Work out the finished part from the listing and answer in its coordinate system (mm). Face numbers are marked on the shaded views. Round coordinates to 2 decimals unless told otherwise and drop trailing zeros. Loops run counter-clockwise (first coordinate to the right, second up) from the corner with the lowest first, then second, coordinate; pieces in that order, holes last. Notation, with made-up numbers: M 40,86.25 L 80,86.25 A9 cw 80,93.25 Z; hole C 68,-37.75 d4. An arc over 180 degrees is marked long. One line per item, written item: value.
```python
from build123d import *

# Parameters (mm, degrees)
SKETCH024_R     = 47.5
PAD007_DEPTH    = 5
SKETCH025_W     = 13.5
SKETCH025_H     = 46
POCKET014_DEPTH = 2.5
SKETCH026_R     = 1.75
POCKET015_DEPTH = 5
SKETCH023_W     = 13.2
SKETCH023_H     = 2.5
PAD008_DEPTH    = 1


with BuildPart() as part:
    # Sketch024 → Pad007 (new body)
    with BuildSketch(Plane.XY):
        Circle(SKETCH024_R)
    extrude(amount=PAD007_DEPTH)

    # Sketch025 (on Face3 of Pad007) → Pocket014 (cut)
    with BuildSketch(Plane.XY.offset(5)):
        Rectangle(SKETCH025_W, SKETCH025_H)
    extrude(amount=-POCKET014_DEPTH, mode=Mode.SUBTRACT)

    # Sketch026 (on Face3 of Pocket014) → Pocket015 (cut)
    with BuildSketch(Plane.XY.offset(5)):
        with Locations((-40, 0)):
            Circle(SKETCH026_R)
        with Locations((-12.363995, 38.041183)):
            Circle(SKETCH026_R)
        with Locations((32.356581, 23.51705)):
            Circle(SKETCH026_R)
        with Locations((32.366826, -23.502949)):
            Circle(SKETCH026_R)
        with Locations((-12.347418, -38.046567)):
            Circle(SKETCH026_R)
    extrude(amount=-POCKET015_DEPTH, mode=Mode.SUBTRACT)

    # Sketch023 (on Face3 of Pocket015) → Pad008 (join)
    with BuildSketch(Plane.XY.offset(5)):
        with Locations((0, 34.25)):
            Rectangle(SKETCH023_W, SKETCH023_H)
    extrude(amount=PAD008_DEPTH)


solid = part.part
```
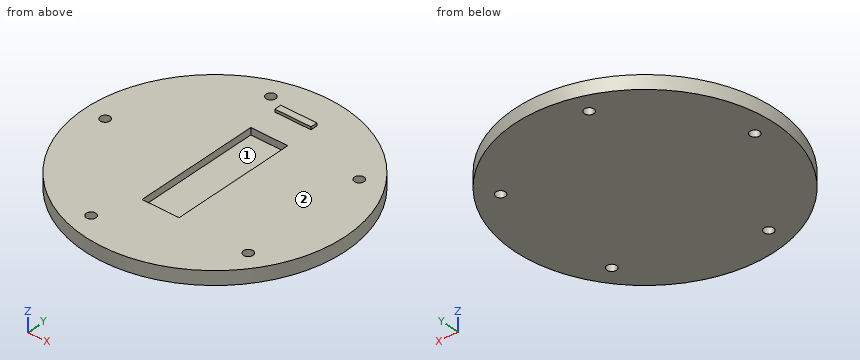
1) Each of these flat-tipped pins is pushed along its axis until it touches: pin 1 (0.8 mm diameter, centred on x = -3, z = 4.5, fed in from +Y); pin 2 (1.2 mm diameter, centred on y = 10.5, z = 3.5, fed in from -X); pin 3 (3 mm diameter, centred on x = 32.37, y = -23.5, fed in from +Z); pin 4 (7 mm diameter, centred on x = 1, y = -1.5, fed in from +Z). Where does it stop, or does it pass through?
Check values:
pin 1: y = 47.43
pin 2: x = -46.46
pin 3: through
pin 4: z = 2.5
2) Find section B-B (x = -40). Give the vertices of the cut face in (y, z), then the cut area to 3 significant figures.
Check values:
outline: M -25.62,0 L -1.75,0 L -1.75,5 L -25.62,5 Z; M 1.75,0 L 25.62,0 L 25.62,5 L 1.75,5 Z
area: 239 mm2
3) The mould has two halves that part along Y. Classify the marked faces 1 and 2: +Y half, -Y half, draft (parallel to the pull), parting line (faces both ways), or undercut.
Check values:
face 1: undercut
face 2: draft
4) Find the intervals of material crossed by probe 1 along Y at (x, z) = (33, 3.75); probe 2 along Z at (x, y) = (-30, -9); probe 3 along Y at (x, z) = (5.5, 5.5), in increasing order. Write a range as from..to.
Check values:
probe 1: -34.17..-25.13, -21.87..21.89, 25.14..34.17
probe 2: 0..5
probe 3: 33..35.5
5) Find section C-C (x = 0). Give the vertices of the cut face in (y, z), then the cut area to 4 significant figures.
Check values:
outline: M -47.5,0 L 47.5,0 L 47.5,5 L 35.5,5 L 35.5,6 L 33,6 L 33,5 L 23,5 L 23,2.5 L -23,2.5 L -23,5 L -47.5,5 Z
area: 362.5 mm2
6) Find section D-D (y = 16). Give the vertices of the cut face in (x, z), then the cut area to 3 significant figures.
Check values:
outline: M -44.72,0 L 44.72,0 L 44.72,5 L 6.75,5 L 6.75,2.5 L -6.75,2.5 L -6.75,5 L -44.72,5 Z
area: 413 mm2
7) Find section A-A (y = 0). Give the vertices of the cut face in (x, z).
Check values:
outline: M -47.5,0 L -41.75,0 L -41.75,5 L -47.5,5 Z; M -38.25,0 L 47.5,0 L 47.5,5 L 6.75,5 L 6.75,2.5 L -6.75,2.5 L -6.75,5 L -38.25,5 Z
